Here's the drawing with two shaded views (mm, measured from the low corner). I have some questions. Round coordinates to 2 decimals unless told otherwise and drop trailing zeros. Write each loop counter-clockwise with the first axis right and the second up, starting at its lowest first coordinate (ties: lowest second). Pieces come first, ordered by that corner, then holes. Notation, with made-up numbers: (82.5, 67) - (109.5, 67) arc R17 cw to (109.5, 80) - close; hole circle Ø4 at (57, 59.5). An arc over 180 degrees is marked (long way). Return JSON: item names as keys, results as strings. Group by question number.
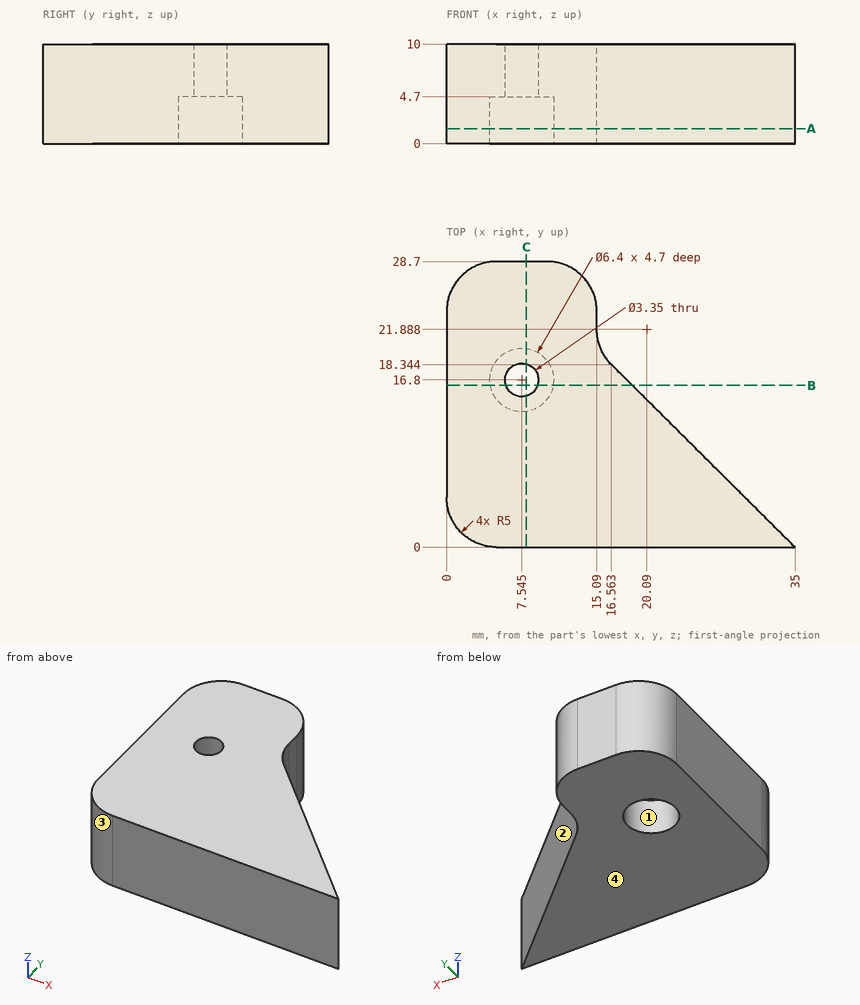
1) If we mould it in two halves opening along Y, with no side actions, what happens to the marked faces 1, 2, 3 and 4? For each: released by +Y, released by -Y, zero draft, split by the parting line, or undercut.
2) I need wall thicknesses on line 1 along X through (y, z) = (21.75, 9.75); line 2 along X through (y, z) = (15.5, 1.25); line 3 along X through (y, z) = (10, 1). Which ranges of each line are inside material? Lowest first, please.
3) Imagine slicing it at A-A (z = 1.5). Please give me the cut outline in (x, y) (1 decimal).
4) Imagine slicing it at B-B (y = 16.25). Please give me the cut outline in (x, z).
5) Imagine slicing it at C-C (x = 8). Please give me the cut outline in (y, z).
6) Will these pins go through, and if not, where does the flat tip stop? pin 1 Ø0.5 at (y, z) = (22.5, 3.5) entering from +X; pin 2 Ø1 at (x, z) = (29, 5.5) entering from +Y.
Results found:
{
 "1": {"face 1": "undercut", "face 2": "released by +Y", "face 3": "released by -Y", "face 4": "zero draft"},
 "2": {"line 1": "x = 0 to 15.09", "line 2": "x = 0 to 4.62, 10.47 to 19.42", "line 3": "x = 0 to 24.95"},
 "3": {"outline": "(0, 5) arc R5 ccw to (5, 0) - (35, 0) - (16.6, 18.3) arc R5 cw to (15.1, 21.9) - (15.1, 23.7) arc R5 ccw to (10.1, 28.7) - (5, 28.7) arc R5 ccw to (0, 23.7) - close; hole circle Ø6.4 at (7.5, 16.8)"},
 "4": {"outline": "(0, 0) - (4.39, 0) - (4.39, 4.7) - (5.96, 4.7) - (5.96, 10) - (0, 10) - close; (9.13, 4.7) - (10.7, 4.7) - (10.7, 0) - (18.67, 0) - (18.67, 10) - (9.13, 10) - close"},
 "5": {"outline": "(0, 0) - (13.63, 0) - (13.63, 4.7) - (15.19, 4.7) - (15.19, 10) - (0, 10) - close; (18.41, 4.7) - (19.97, 4.7) - (19.97, 0) - (28.7, 0) - (28.7, 10) - (18.41, 10) - close"},
 "6": {"pin 1": "stops at x = 15.09", "pin 2": "stops at y = 6.47"}
}
